Can you work these out from the model? Positions are in its coordinate system, mm. Face numbers are marked on the shaded views. A direction names the side the tool comes from. Coordinates: 2 decimals unless noted, no trailing zeros. Order: outer loops, then holes, each group sorted by start corner. A loop starts at its lowest first (then second) coordinate and runs counter-clockwise, first axis right, second up. Notation, with made-up numbers: (-26, 41.5) -> (16, 41.5) arc R18 ccw to (16, 55.5) -> close; hole circle Ø11 at (21.25, 54). An arc over 180 degrees is marked (long way). Answer in a Markdown table with one row per item. Add a question column.
1. Imagine slicing it at A-A on x = 0. Write out the boundary of the cut face in (y, z), plus the area to 3 significant figures.
2. If I drill on line 1 along Y through (x, z) = (0, 2.5); line 2 along Y through (x, z) = (0, 10.25); line 3 along Z through (x, y) = (-10, -2), over which ranges is the centre line in solid material (lowest first)? Write a range as [from, to].
3. Imagine slicing it at D-D on z = 9.5. Write out the boundary of the cut face in (x, y), plus the area to 3 significant figures.
4. Imagine slicing it at B-B on z = 5.5. Write out the boundary of the cut face in (x, y).
5. Will these pins go through, and if not, where does the flat tip stop? pin 1 (1.5 mm diameter, centred on y = 0.5, z = 6.5, fed in from +X); pin 2 (4 mm diameter, centred on x = 0, y = -9, fed in from +Z); pin 3 (5 mm diameter, centred on y = 5, z = 14.5, fed in from -X).
6. On a 3-axis mill with a long thin cutter (end or side, diameter ignored), from which of +Z, -Z, +X, -X, +Y, -Y can I reach the whole of each face in a straight line? I mean the marked faces 1 and 2. Say none if no direction works.
7. Imagine slicing it at C-C on y = 9. Write out the boundary of the cut face in (x, z).
8. We'd pull the mould along Y, two halves only. Please class the marked faces 3, 4 and 5: pulls with the +Y half, pulls with the -Y half, needs draft (parallel to the pull), parting line crosses it, or undercut.
from build123d import *

# Parameters (mm, degrees)
SKETCH1_R           = 13.75
BOSS_EXTRUDE1_DEPTH = 16
SKETCH2_R           = 11.75
CUT_EXTRUDE1_DEPTH  = 8
SKETCH3_R           = 1.75
CUT_EXTRUDE2_DEPTH  = 26.181838694
SKETCH4_R           = 2
CUT_EXTRUDE4_DEPTH  = 26.181838694


with BuildPart() as part:
    # Sketch1 → Boss-Extrude1 (new body)
    with BuildSketch(Plane(origin=(0, 0, 0), x_dir=(0, 1, 0), z_dir=(0, 0, 1))):
        with Locations(Location((0, 0, 0), (0, 0, 270))):
            Circle(SKETCH1_R)
    extrude(amount=BOSS_EXTRUDE1_DEPTH)

    # Sketch2 → Cut-Extrude1 (cut)
    with BuildSketch(Plane(origin=(0, 0, 16), x_dir=(0, -1, 0), z_dir=(0, 0, 1))):
        with Locations(Location((0, 0, 0), (0, 0, 90))):
            Circle(SKETCH2_R)
    extrude(amount=-CUT_EXTRUDE1_DEPTH, mode=Mode.SUBTRACT)

    # Sketch3 → Cut-Extrude2 (cut, through all)
    with BuildSketch(Plane(origin=(0, 0, 0), x_dir=(1, 0, 0), z_dir=(0, 0, -1))):
        with Locations(Location((0, 9, 0), (0, 0, 180))):
            Circle(SKETCH3_R)
        with Locations(Location((0, -9, 0), (0, 0, 180))):
            Circle(SKETCH3_R)
    extrude(amount=-CUT_EXTRUDE2_DEPTH, mode=Mode.SUBTRACT)

    # Sketch4 → Cut-Extrude4 (cut, through all)
    with BuildSketch(Plane(origin=(0, 0, 0), x_dir=(1, 0, 0), z_dir=(0, 0, -1))):
        with Locations((-14, 0)):
            Circle(SKETCH4_R)
    cut_extrude4 = extrude(amount=-CUT_EXTRUDE4_DEPTH, mode=Mode.SUBTRACT)

    # Mirror1: Cut-Extrude4 across plane
    add(cut_extrude4.mirror(Plane(origin=(0, 0, 0), x_dir=(0, 0, 1), z_dir=(1, 0, 0))), mode=Mode.SUBTRACT)


solid = part.part
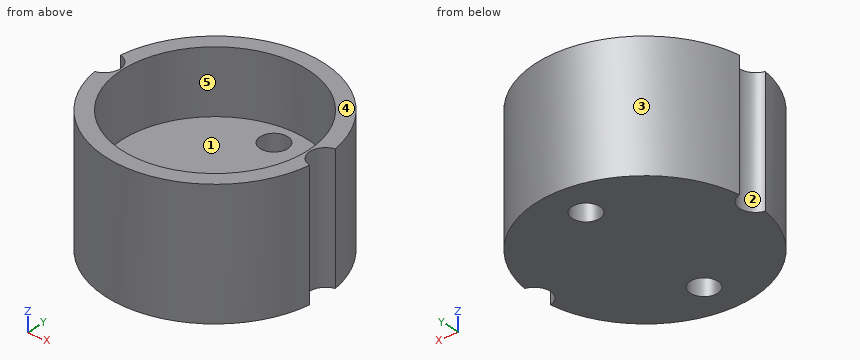
Answers follow:
| question | item | result |
|---|---|---|
| 1 | outline | (-13.75, 0) -> (-10.75, 0) -> (-10.75, 8) -> (-11.75, 8) -> (-11.75, 16) -> (-13.75, 16) -> close; (-7.25, 0) -> (7.25, 0) -> (7.25, 8) -> (-7.25, 8) -> close; (10.75, 0) -> (13.75, 0) -> (13.75, 16) -> (11.75, 16) -> (11.75, 8) -> (10.75, 8) -> close |
| 1 | area | 196 mm² |
| 2 | line 1 | y = [-13.75, -10.75], [-7.25, 7.25], [10.75, 13.75] |
| 2 | line 2 | y = [-13.75, -11.75], [11.75, 13.75] |
| 2 | line 3 | z = [0, 8] |
| 3 | outline | (-13.61, -1.96) arc R13.75 ccw to (13.61, -1.96) arc R2 cw to (13.61, 1.96) arc R13.75 ccw to (-13.61, 1.96) arc R2 cw to start; hole circle Ø23.5 at (0, 0) |
| 3 | area | 150 mm² |
| 4 | outline | (-13.61, -1.96) arc R13.75 ccw to (13.61, -1.96) arc R2 cw to (13.61, 1.96) arc R13.75 ccw to (-13.61, 1.96) arc R2 cw to start; hole circle Ø3.5 at (0, -9); hole circle Ø3.5 at (0, 9) |
| 5 | pin 1 | stops at x = 12.44 |
| 5 | pin 2 | stops at z = 8 |
| 5 | pin 3 | stops at x = -13.52 |
| 6 | face 1 | +Z |
| 6 | face 2 | +Z, -Z, -X |
| 7 | outline | (-10.4, 0) -> (-1.75, 0) -> (-1.75, 8) -> (-7.55, 8) -> (-7.55, 16) -> (-10.4, 16) -> close; (1.75, 0) -> (10.4, 0) -> (10.4, 16) -> (7.55, 16) -> (7.55, 8) -> (1.75, 8) -> close |
| 8 | face 3 | pulls with the +Y half |
| 8 | face 4 | needs draft |
| 8 | face 5 | undercut |
